Geometry check sheet. Reference: the model listing, model coordinates, mm. A direction names the side the tool comes from. Round coordinates to 2 decimals unless told otherwise and drop trailing zeros. Write each loop counter-clockwise with the first axis right and the second up, starting at its lowest first coordinate (ties: lowest second). Pieces come first, ordered by that corner, then holes. Notation, with made-up numbers: (-22, -39.75) - (32, -39.75) arc R18 ccw to (32, -35.75) - close; hole circle Ø9 at (15.5, 7.5). An arc over 180 degrees is marked (long way). Return JSON: item names as keys, results as strings.
```python
from build123d import *

# Parameters (mm, degrees)
F0_R     = 1.375
F1_DEPTH = 1.6
F2_W     = 8.457642
F2_H     = 1.740684
F2_H_2   = 4.566714
F3_DEPTH = 4
F4_W     = 20
F4_H     = 15
F4_W_2   = 23
F4_H_2   = 18
F5_DEPTH = 17
F6_W     = 15
F6_H     = 12.5
F7_DEPTH = 6


with BuildPart() as f1:
    # F0 (on Top) → F1 (new body)
    with BuildSketch(Plane.XY):
        with BuildLine():
            Line((-39.5, -28), (39.5, -28))
            ThreePointArc((39.5, -28), (41.62132, -27.12132), (42.5, -25))
            Line((42.5, -25), (42.5, 25))
            ThreePointArc((42.5, 25), (41.62132, 27.12132), (39.5, 28))
            Line((39.5, 28), (-39.5, 28))
            ThreePointArc((-39.5, 28), (-41.62132, 27.12132), (-42.5, 25))
            Line((-42.5, 25), (-42.5, -25))
            ThreePointArc((-42.5, -25), (-41.62132, -27.12132), (-39.5, -28))
        make_face()
        with Locations((-39, -24.5)):
            Circle(F0_R, mode=Mode.SUBTRACT)
        with Locations((19, -24.5)):
            Circle(F0_R, mode=Mode.SUBTRACT)
        with Locations((-39, 24.5)):
            Circle(F0_R, mode=Mode.SUBTRACT)
        with Locations((19, 24.5)):
            Circle(F0_R, mode=Mode.SUBTRACT)
    extrude(amount=F1_DEPTH)

    # F2 (on face) → F3 (join)
    with BuildSketch(Plane.XY.offset(1.6)):
        with Locations((-31.9, -28.870342)):
            Rectangle(F2_W, F2_H)
        with Locations((-31.9, -25.716643)):
            Rectangle(F2_W, F2_H_2)
    extrude(amount=F3_DEPTH)

    # F4 (on face) → F5 (join)
    with BuildSketch(Plane.XY.offset(1.6)):
        with Locations((34.5, 19)):
            Rectangle(F4_W, F4_H)
        with Locations((34.5, 1)):
            Rectangle(F4_W, F4_H)
        with Locations((33, -17.75)):
            Rectangle(F4_W_2, F4_H_2)
    extrude(amount=F5_DEPTH)

    # F6 (on face) → F7 (join)
    with BuildSketch(Plane.XY.offset(1.6)):
        with Locations((-10.5, -23.75)):
            Rectangle(F6_W, F6_H)
    extrude(amount=F7_DEPTH)


solid = f1.part
```
(1) Material ranges on line 1 along Y through (x, z) = (27, 5.5); line 2 along Y through (x, z) = (19, 0.95) (3 decimals); line 3 along X through (y, z) = (6, 6.75), recorded low to high. Write a range as [from, to].
Response values:
{"line 1": "y = [-26.75, -8.75], [-6.5, 8.5], [11.5, 26.5]", "line 2": "y = [-28, -25.875], [-23.125, 23.125], [25.875, 28]", "line 3": "x = [24.5, 44.5]"}
(2) Release check for a two-part mould opening along Y. For faces 4 (the face through (-1, 0, 0)), 5 (the face through (17.987, -23.571, 0.789)), 6 (the face through (-41.64, -27.1, 0.79)) record: pulls with the +Y half, pulls with the -Y half, needs draft (parallel to the pull), parting line crosses it, or undercut.
Response values:
{"face 4": "needs draft", "face 5": "undercut", "face 6": "pulls with the -Y half"}
(3) Section check D-D, the plane y = -1. Enter the section's corners in (x, z).
Response values:
{"outline": "(-42.5, 0) - (42.5, 0) - (42.5, 1.6) - (44.5, 1.6) - (44.5, 18.6) - (24.5, 18.6) - (24.5, 1.6) - (-42.5, 1.6) - close"}
(4) Section check C-C, the plane y = -19. Enter the section's corners in (x, z), plus the area to 3 significant figures.
Response values:
{"outline": "(-42.5, 0) - (42.5, 0) - (42.5, 1.6) - (44.5, 1.6) - (44.5, 18.6) - (21.5, 18.6) - (21.5, 1.6) - (-3, 1.6) - (-3, 7.6) - (-18, 7.6) - (-18, 1.6) - (-42.5, 1.6) - close", "area": "617 mm^2"}
(5) Gauge pin test, flat ends, axial feed: pin 1 (5 mm diameter, centred on x = 38, z = 13.5, fed in from +Y); pin 2 (5 mm diameter, centred on x = -24.5, y = -0.5, fed in from -Z); pin 3 (6 mm diameter, centred on x = -12.5, y = -23, fed in from +Z); pin 4 (8.5 mm diameter, centred on y = -20.5, z = 6, fed in from -X). Record the tip position at first contact, or that the pin passes through.
Response values:
{"pin 1": "stops at y = 26.5", "pin 2": "stops at z = 0", "pin 3": "stops at z = 7.6", "pin 4": "stops at x = -36.13"}
(6) Section check B-B, the plane x = -32.5. Enter the section's corners in (y, z), plus the area to 3 significant figures.
Response values:
{"outline": "(-29.74, 1.6) - (-28, 1.6) - (-28, 0) - (28, 0) - (28, 1.6) - (-23.43, 1.6) - (-23.43, 5.6) - (-29.74, 5.6) - close", "area": "115 mm^2"}
(7) Access from +Z, -Z, +X, -X, +Y, -Y to the whole of each face (thin tool, end or side, straight path). Record for faces 1 (the face through (-27.671, -27, 4)), 2 (the face through (-32, -29.741, 4)), 3 (the face through (-11, -29, 1.6)).
Response values:
{"face 1": "+Z, +Y, -Y", "face 2": "+Z, -Z, -X, -Y", "face 3": "-Z, +X, -X, -Y"}
(8) Section check A-A, the plane x = 19. Enter the section's corners in (y, z) (3 decimals), plus the area to 3 significant figures.
Response values:
{"outline": "(-28, 0) - (-25.875, 0) - (-25.875, 1.6) - (-28, 1.6) - close; (-23.125, 0) - (23.125, 0) - (23.125, 1.6) - (-23.125, 1.6) - close; (25.875, 0) - (28, 0) - (28, 1.6) - (25.875, 1.6) - close", "area": "80.8 mm^2"}
